Geometry: final body of the model. Coordinates: model frame, mm. Face numbers are marked on the shaded views. A direction names the side the tool comes from. Give positions to 0.01 mm unless a question says otherwise; leave off trailing zeros. Order: outer loops, then holes, each group sorted by start corner. A loop starts at its lowest first (then second) coordinate and runs counter-clockwise, first axis right, second up. Notation, with made-up numbers: (-20.5, 17.5) -> (15.5, 17.5) arc R16 cw to (15.5, 43.5) -> close; hole circle Ø4 at (8, -21). An arc over 180 degrees is marked (long way). One line per question, with ' | ' between items. Start each with the question number.
(1) Mould query, pull axis X, two halves, no side actions, for the marked faces 1, 2, 3 and 4. Classes: +X half, -X half, draft (parallel to the pull), parting line (faces both ways), or undercut.
(2) Section D-D (y = 26.5). Return loops of the section in (x, z).
(3) Set-up query: the marked faces 5, 6, 7, 8 and 9. Return all of +Z, -Z, +X, -X, +Y, -Y with unobstructed straight access to the full face (end or side cutting, diameter ignored); none if empty.
(4) Section B-B (z = 33). Return loops of the section in (x, y).
(5) Section C-C (x = 18). Return loops of the section in (y, z).
(6) First-contact query: pin 1 Ø1.5 at (x, z) = (16.5, 31.5) entering from -Y; pin 2 Ø3 at (x, y) = (-9, -15.5) entering from -Z; pin 3 Ø12 at (x, y) = (1, -16) entering from +Z. Flat tips, straight axial feed; report the tip coordinate or a pass-through.
(7) Ray query, L1, parallel to X at y = 20.5, z = 33; L2, parallel to X at y = -12.5, z = 29; L3, parallel to Z at x = 17.5, y = 22.25. Return the intervals inside material, ascending.
(8) Section A-A (y = -9). Return loops of the section in (x, z).
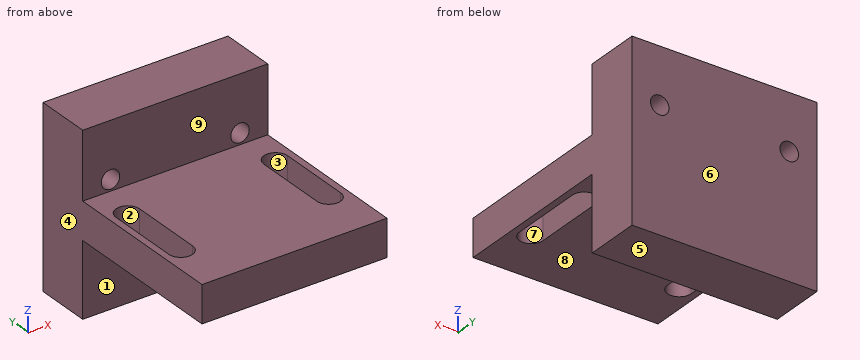
```python
from build123d import *

# Parameters (mm, degrees)
SKETCH_1_W             = 50
SKETCH_1_H             = 60
EXTRUDE_1_DEPTH        = 30
SKETCH_2_W             = 50
SKETCH_2_H             = 45
CUT_EXTRUDE_1_DEPTH    = 20
CUT_EXTRUDE_2_DEPTH    = 11
SKETCH_6_W             = 50
SKETCH_6_H             = 15
EXTRUDE_2_DEPTH        = 18
HOLE_WIZARD_M6_1_D     = 5
HOLE_WIZARD_M6_1_DEPTH = 15
HOLE_WIZARD_M6_1_TIP   = 1.502151548


with BuildPart() as part:
    # 草图1 → 凸台-拉伸1 (new body)
    with BuildSketch(Plane.XY):
        Rectangle(SKETCH_1_W, SKETCH_1_H)
    extrude(amount=EXTRUDE_1_DEPTH)

    # 草图2 → 切除-拉伸1 (cut)
    with BuildSketch(Plane(origin=(0, 0, 0), x_dir=(-1, 0, 0), z_dir=(0, 0, -1))):
        with Locations((0, -7.5)):
            Rectangle(SKETCH_2_W, SKETCH_2_H)
    extrude(amount=-CUT_EXTRUDE_1_DEPTH, mode=Mode.SUBTRACT)

    # 草图3 → 切除-拉伸2 (cut, through all)
    with BuildSketch(Plane(origin=(0, 0, 20), x_dir=(-1, 0, 0), z_dir=(0, 0, -1))):
        with BuildLine():
            Line((-23.2, -15), (-23.2, 5))
            ThreePointArc((-23.2, 5), (-20, 8.2), (-16.8, 5))
            Line((-16.8, 5), (-16.8, -15))
            ThreePointArc((-16.8, -15), (-20, -18.2), (-23.2, -15))
        make_face()
        with BuildLine():
            Line((23.2, -15), (23.2, 5))
            ThreePointArc((23.2, 5), (20, 8.2), (16.8, 5))
            Line((16.8, 5), (16.8, -15))
            ThreePointArc((16.8, -15), (20, -18.2), (23.2, -15))
        make_face()
    extrude(amount=-CUT_EXTRUDE_2_DEPTH, mode=Mode.SUBTRACT)

    # 草图6 → 凸台-拉伸2 (add)
    with BuildSketch(Plane.XY.offset(30)):
        with Locations((0, 22.5)):
            Rectangle(SKETCH_6_W, SKETCH_6_H)
    extrude(amount=EXTRUDE_2_DEPTH)

    # M6 螺纹孔1
    with Locations(Plane(origin=(17.5, 30, 33), x_dir=(1, 0, 0), z_dir=(0, 1, 0))):
        with Locations((0, 0), (-35, 0)):
            Hole(HOLE_WIZARD_M6_1_D / 2, depth=HOLE_WIZARD_M6_1_DEPTH)
            with Locations((0, 0, -(HOLE_WIZARD_M6_1_DEPTH + HOLE_WIZARD_M6_1_TIP / 2))):  # 118° drill point
                Cone(0, HOLE_WIZARD_M6_1_D / 2, HOLE_WIZARD_M6_1_TIP, mode=Mode.SUBTRACT)


solid = part.part
```
Response:
1) face 1: draft | face 2: undercut | face 3: undercut | face 4: -X half
2) outline: (-25, 0) -> (25, 0) -> (25, 48) -> (-25, 48) -> close; hole circle Ø5 at (-17.5, 33); hole circle Ø5 at (17.5, 33)
3) face 5: -Z, +X, -X, +Y, -Y | face 6: +Z, -Z, +X, -X, +Y | face 7: +Z, -Z | face 8: -Z, +X, -X, -Y | face 9: +Z, +X, -X, -Y
4) outline: (-25, 15) -> (-20, 15) -> (-20, 30) -> (-25, 30) -> close; (-15, 15) -> (15, 15) -> (15, 30) -> (-15, 30) -> close; (20, 15) -> (25, 15) -> (25, 30) -> (20, 30) -> close
5) outline: (-30, 20) -> (-17.5, 20) -> (-17.5, 30) -> (-30, 30) -> close; (7.5, 20) -> (15, 20) -> (15, 0) -> (30, 0) -> (30, 30.55) -> (15, 30.55) -> (15, 30) -> (7.5, 30) -> close; (15, 35.45) -> (30, 35.45) -> (30, 48) -> (15, 48) -> close
6) pin 1: stops at y = 15 | pin 2: stops at z = 20 | pin 3: stops at z = 30
7) L1: x = -25 to -20, -15 to 15, 20 to 25 | L2: x = -25 to -23.2, -16.8 to 16.8, 23.2 to 25 | L3: z = 0 to 30.5, 35.5 to 48
8) outline: (-25, 20) -> (-23.2, 20) -> (-23.2, 30) -> (-25, 30) -> close; (-16.8, 20) -> (16.8, 20) -> (16.8, 30) -> (-16.8, 30) -> close; (23.2, 20) -> (25, 20) -> (25, 30) -> (23.2, 30) -> close
